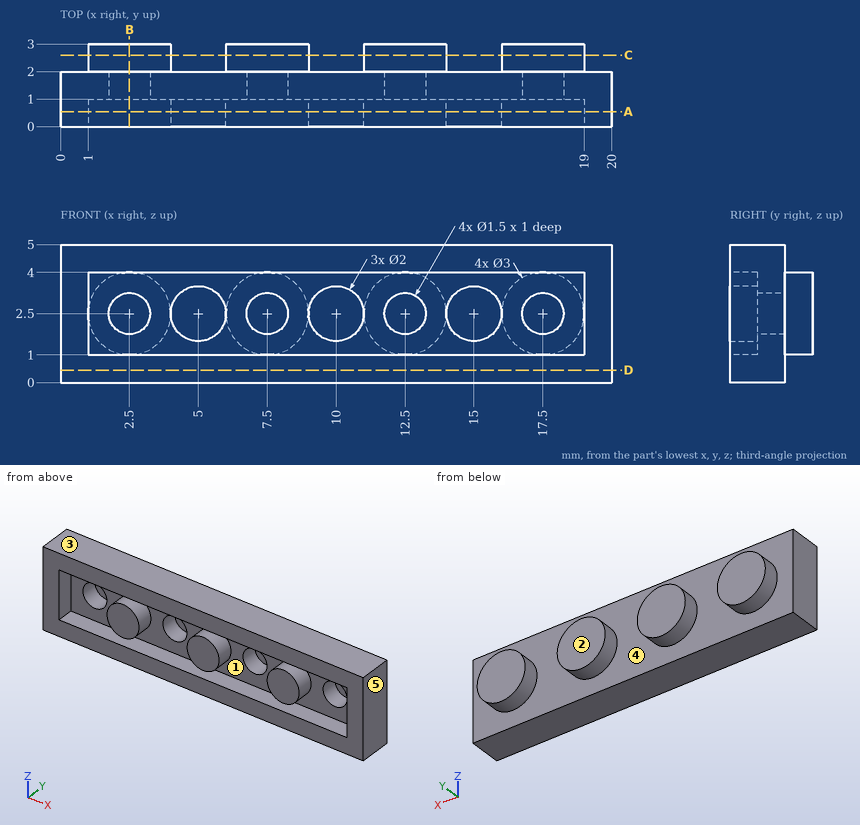
Answer from the drawing. Dimensions are ordinates in mm from the lowest x, y and z of the part. A direction names the side the tool comes from. Give positions to 0.01 mm unless a question says otherwise; leave off trailing zeros. Order: outer loops, then holes, each group sorted by start corner. A loop starts at its lowest first (then second) coordinate and runs counter-clockwise, first axis right, second up.
(1) Given pin 1 (0.5 mm diameter, centred on x = 11.5, y = 0.5, fed in from -Z); pin 2 (2.5 mm diameter, centred on x = 7.5, z = 2.5, fed in from -Y), each flat-ended and moving along its own axis, determine where each tip first touches the part or whether it passes through.
(2) Find section A-A (y = 0.55). Give the vertices of the cut face in (x, z), plus the area to 3 significant figures.
(3) For the marked faces 4 and 5, determine the directions among +Z, -Z, +X, -X, +Y, -Y from which every point of the face is accessible in a straight line to the end or side of a thin tool.
(4) Find section D-D (z = 0.45). Give the vertices of the cut face in (x, y), plus the area to 3 significant figures.
(5) For a pull along Z with two mould halves and no side action, classify the marked faces 1, 2 and 3 as released by +Z, released by -Z, zero draft, split by the parting line, or undercut.
(6) Find section C-C (y = 2.6). Give the vertices of the cut face in (x, z), plus the area to 3 significant figures.
(7) Straight lines are drawn through the part: L1, parallel to X at y = 1.6, z = 2.5; L2, parallel to X at y = 2.5, z = 3.8; L3, parallel to Y at x = 18.5, z = 1.8. For each, find the intervals that lie inside material, in ascending order.
(8) Find section B-B (x = 2.5). Give the vertices of the cut face in (y, z), plus the area to 3 significant figures.
Result sheet:
1. pin 1: stops at z = 0
1. pin 2: stops at y = 1
2. outline: (0, 0) - (20, 0) - (20, 5) - (0, 5) - close; circle Ø2 at (5, 2.5); circle Ø2 at (10, 2.5); circle Ø2 at (15, 2.5); hole (1, 1) - (19, 1) - (19, 4) - (1, 4) - close
2. area: 55.4 mm2
3. face 4: +Y
3. face 5: +Z, -Z, +X, +Y, -Y
4. outline: (0, 0) - (20, 0) - (20, 2) - (0, 2) - close
4. area: 40.0 mm2
5. face 1: undercut
5. face 2: zero draft
5. face 3: released by +Z
6. outline: circle Ø3 at (2.5, 2.5); circle Ø3 at (7.5, 2.5); circle Ø3 at (12.5, 2.5); circle Ø3 at (17.5, 2.5)
6. area: 28.3 mm2
7. L1: x = 0 to 1.75, 3.25 to 6.75, 8.25 to 11.75, 13.25 to 16.75, 18.25 to 20
7. L2: x = 1.75 to 3.25, 6.75 to 8.25, 11.75 to 13.25, 16.75 to 18.25
7. L3: y = 1 to 3
8. outline: (0, 0) - (2, 0) - (2, 1) - (3, 1) - (3, 4) - (2, 4) - (2, 5) - (0, 5) - (0, 4) - (1, 4) - (1, 3.25) - (2, 3.25) - (2, 1.75) - (1, 1.75) - (1, 1) - (0, 1) - close
8. area: 8.50 mm2
